Can you work these out from the model? Positions are in its coordinate system, mm. A direction names the side the tool comes from. Coordinates: 2 decimals unless noted, no trailing zeros. Put each result on its own line as item: value. Start each with the question number.
Item 1: For faces 4 (the cylindrical face through (5.37, 2.46, 15.77)), 5 (the cylindrical face through (7.179, 1.014, -31.696)), 6 (the cylindrical face through (-0.3, 12.021, 14.546)), which set-ups out of +Z, -Z, +X, -X, +Y, -Y let a thin tool reach every point of the face, with its end or its side?
Item 2: We'd pull the mould along Z, two halves only. Please class faces 1 (the cylindrical face through (-12.58, 12.02, 8.29)), 2 (the flat face through (-10, 5, -12)), 3 (the cylindrical face through (-33.787, 3.042, -9.133)): pulls with the +Z half, pulls with the -Z half, needs draft (parallel to the pull), parting line crosses it, or undercut.
Item 3: If we section it at B-B on z = 0: State how many separate pieces and enclosed holes the cut face has, plus the area to 4 significant figures.
Item 4: Will these pins go through, and if not, where does the flat tip stop? P1, Ø2.5, axis at x = -30.43, z = -8.15, coming from the +Y side; P2, Ø2, axis at y = 5, z = -26.5, coming from the +X side; P3, Ø6, axis at y = 5.5, z = 16, coming from the -X side; P4, Ø3, axis at y = 6, z = 16.5, coming from the -X side.
Item 5: Please list where these lines run through material, in increasing order: L1, parallel to Z at x = -5.5, y = 3.5; L2, parallel to Z at x = 6.5, y = 8.5; L3, parallel to X at y = 12.25, z = -8. Write a range as from..to.
```python
from build123d import *

# Parameters (mm, degrees)
SKETCH1_R           = 28
BOSS_EXTRUDE1_DEPTH = 6
SKETCH2_R           = 19
BOSS_EXTRUDE2_DEPTH = 0.5
SKETCH3_R           = 17.5
BOSS_EXTRUDE3_DEPTH = 7
SKETCH4_R           = 1
CUT_EXTRUDE1_DEPTH  = 3
CIRPATTERN1_COUNT   = 6
SKETCH5_R           = 11.5
CUT_EXTRUDE2_DEPTH  = 4
SKETCH6_R           = 10
CUT_EXTRUDE3_DEPTH  = 9.5
SKETCH7_R           = 1.6
CUT_EXTRUDE4_DEPTH  = 13.5
SKETCH9_R           = 3.5
CUT_EXTRUDE10_DEPTH = 5
SKETCH10_R          = 2
CUT_EXTRUDE11_DEPTH = 11
CIRPATTERN2_COUNT   = 6
CHAMFER1_SIZE       = 1
CHAMFER2_SIZE       = 0.5
SKETCH13_R          = 1.6
BOSS_EXTRUDE4_DEPTH = 6
SKETCH14_R          = 2
CUT_EXTRUDE12_DEPTH = 4
CIRPATTERN3_COUNT   = 4


with BuildPart() as part:
    # Sketch1 → Boss-Extrude1 (new body)
    with BuildSketch(Plane(origin=(0, 0, 0), x_dir=(1, 0, 0), z_dir=(0, 1, 0))):
        with Locations(Location((0, 0, 0), (0, 0, 270))):
            Circle(SKETCH1_R)
    extrude(amount=BOSS_EXTRUDE1_DEPTH)

    # Sketch2 → Boss-Extrude2 (add)
    with BuildSketch(Plane(origin=(0, 6, 0), x_dir=(1, 0, 0), z_dir=(0, 1, 0))):
        with Locations(Location((0, 0, 0), (0, 0, 270))):
            Circle(SKETCH2_R)
    extrude(amount=BOSS_EXTRUDE2_DEPTH)

    # Sketch3 → Boss-Extrude3 (add)
    with BuildSketch(Plane(origin=(0, 6.5, 0), x_dir=(1, 0, 0), z_dir=(0, 1, 0))):
        with Locations(Location((0, 0, 0), (0, 0, 270))):
            Circle(SKETCH3_R)
    extrude(amount=BOSS_EXTRUDE3_DEPTH)

    # Sketch4 → Cut-Extrude1 (cut)
    with BuildSketch(Plane(origin=(0, 13.5, 0), x_dir=(1, 0, 0), z_dir=(0, 1, 0))):
        with Locations(Location((0, 15.5, 0), (0, 0, 270))):
            Circle(SKETCH4_R)
    cut_extrude1 = extrude(amount=-CUT_EXTRUDE1_DEPTH, mode=Mode.SUBTRACT)

    # CirPattern1: Cut-Extrude1 ×6 about axis
    cirpattern1_axis = Axis((0, 0, 0), (0, 1, 0))
    for i in range(1, CIRPATTERN1_COUNT):
        add(cut_extrude1.rotate(cirpattern1_axis, i * 360 / CIRPATTERN1_COUNT), mode=Mode.SUBTRACT)

    # Sketch5 → Cut-Extrude2 (cut)
    with BuildSketch(Plane(origin=(0, 13.5, 0), x_dir=(1, 0, 0), z_dir=(0, 1, 0))):
        with Locations(Location((0, 0, 0), (0, 0, 270))):
            Circle(SKETCH5_R)
    extrude(amount=-CUT_EXTRUDE2_DEPTH, mode=Mode.SUBTRACT)

    # Sketch6 → Cut-Extrude3 (cut)
    with BuildSketch(Plane(origin=(0, 9.5, 0), x_dir=(1, 0, 0), z_dir=(0, 1, 0))):
        with Locations(Location((0, 0, 0), (0, 0, 270))):
            Circle(SKETCH6_R)
    extrude(amount=-CUT_EXTRUDE3_DEPTH, mode=Mode.SUBTRACT)

    # Sketch7 → Cut-Extrude4 (cut)
    with BuildSketch(Plane(origin=(0, 13.5, 0), x_dir=(1, 0, 0), z_dir=(0, 1, 0))):
        with Locations(Location((7.5, 12.990381057, 0), (0, 0, 270))):
            Circle(SKETCH7_R)
    cut_extrude4 = extrude(amount=-CUT_EXTRUDE4_DEPTH, mode=Mode.SUBTRACT)

    # Sketch9 → Cut-Extrude10 (cut)
    with BuildSketch(Plane.XZ):
        with Locations(Location((7.5, -12.990381057, 0), (0, 0, 270))):
            Circle(SKETCH9_R)
    cut_extrude10 = extrude(amount=-CUT_EXTRUDE10_DEPTH, mode=Mode.SUBTRACT)

    # Sketch10 → Cut-Extrude11 (cut)
    with BuildSketch(Plane.XZ):
        with Locations(Location((7.5, -12.990381057, 0), (0, 0, 270))):
            Circle(SKETCH10_R)
    cut_extrude11 = extrude(amount=-CUT_EXTRUDE11_DEPTH, mode=Mode.SUBTRACT)

    # CirPattern2: Cut-Extrude4, Cut-Extrude10, Cut-Extrude11 ×6 about axis
    cirpattern2_axis = Axis((0, 0, 0), (0, 1, 0))
    add([cut_extrude4.rotate(cirpattern2_axis, i * 360 / CIRPATTERN2_COUNT) for i in range(1, CIRPATTERN2_COUNT)], mode=Mode.SUBTRACT)
    add([cut_extrude10.rotate(cirpattern2_axis, i * 360 / CIRPATTERN2_COUNT) for i in range(1, CIRPATTERN2_COUNT)], mode=Mode.SUBTRACT)
    add([cut_extrude11.rotate(cirpattern2_axis, i * 360 / CIRPATTERN2_COUNT) for i in range(1, CIRPATTERN2_COUNT)], mode=Mode.SUBTRACT)

    # Chamfer1
    chamfer1_edges = [part.edges().sort_by_distance(p)[0] for p in [
        (0, 0, -10),
    ]]
    chamfer(chamfer1_edges, length=CHAMFER1_SIZE)

    # Chamfer2
    chamfer2_edges = [part.edges().sort_by_distance(p)[0] for p in [
        (0, 13.5, -17.5),
        (0, 13.5, -11.5),
    ]]
    chamfer(chamfer2_edges, length=CHAMFER2_SIZE)

    # Sketch13 → Boss-Extrude4 (add)
    with BuildSketch(Plane(origin=(0, 6, 0), x_dir=(1, 0, 0), z_dir=(0, 1, 0))):
        with BuildLine():
            Line((4.772059529, 31.332530186), (3.027664457, 24.822359149))
            Line((3.027664457, 24.822359149), (9.789145241, 23.010625833))
            Line((9.789145241, 23.010625833), (11.533540313, 29.52079687))
            ThreePointArc((11.533540313, 29.52079687), (9.058666579, 33.80740392), (4.772059529, 31.332530186))
        make_face()
        with Locations(Location((8.152799921, 30.426663528, 0), (0, 0, 270))):
            Circle(SKETCH13_R, mode=Mode.SUBTRACT)
    boss_extrude4 = extrude(amount=-BOSS_EXTRUDE4_DEPTH)

    # Sketch14 → Cut-Extrude12 (cut)
    with BuildSketch(Plane(origin=(0, 6, 0), x_dir=(1, 0, 0), z_dir=(0, 1, 0))):
        with Locations(Location((8.152799921, 30.426663528, 0), (0, 0, 270))):
            Circle(SKETCH14_R)
    cut_extrude12 = extrude(amount=-CUT_EXTRUDE12_DEPTH, mode=Mode.SUBTRACT)

    # CirPattern3: Boss-Extrude4, Cut-Extrude12 ×4 about axis
    cirpattern3_axis = Axis((0, 0, 0), (0, 1, 0))
    add([boss_extrude4.rotate(cirpattern3_axis, i * 360 / CIRPATTERN3_COUNT) for i in range(1, CIRPATTERN3_COUNT)])
    add([cut_extrude12.rotate(cirpattern3_axis, i * 360 / CIRPATTERN3_COUNT) for i in range(1, CIRPATTERN3_COUNT)], mode=Mode.SUBTRACT)


solid = part.part
```
Solutions:
1. face 4: -Y
1. face 5: +Y, -Y
1. face 6: +Y
2. face 1: undercut
2. face 2: undercut
2. face 3: parting line crosses it
3. separate pieces: 4
3. enclosed holes: 0
3. area: 182.5 mm^2
4. P1: through
4. P2: x = 11.57
4. P3: x = -24.8
4. P4: x = -23.64
5. L1: -27.45..-15.86, -10.12..-8.35, 8.35..10.12, 15.86..32.71
5. L2: -16.25..-14.72, -11.26..-7.6, 7.6..11.26, 14.72..16.25
5. L3: -15.56..-14.39, -12.46..-8.26, 8.26..12.46, 14.39..15.56
